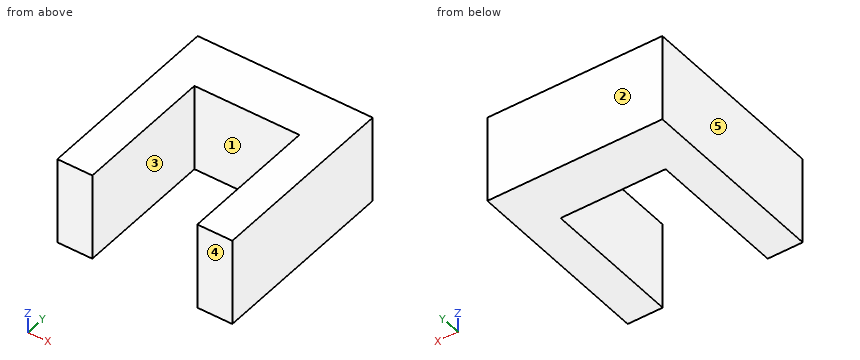
```python
from build123d import *

# Parameters (mm, degrees)
SKETCH1_W           = 50
SKETCH1_H           = 15
BOSS_EXTRUDE1_DEPTH = 25
SKETCH2_W           = 10
SKETCH2_H           = 41
BOSS_EXTRUDE2_DEPTH = 25
SKETCH3_W           = 10
SKETCH3_H           = 41
BOSS_EXTRUDE3_DEPTH = 25


with BuildPart() as part:
    # Sketch1 → Boss-Extrude1 (new body)
    with BuildSketch(Plane.XY):
        with Locations((0, 7.5)):
            Rectangle(SKETCH1_W, SKETCH1_H)
    extrude(amount=BOSS_EXTRUDE1_DEPTH)

    # Sketch2 → Boss-Extrude2 (add)
    with BuildSketch(Plane.XY):
        with Locations((-20, -19.5)):
            Rectangle(SKETCH2_W, SKETCH2_H)
    extrude(amount=BOSS_EXTRUDE2_DEPTH)

    # Sketch3 → Boss-Extrude3 (add)
    with BuildSketch(Plane.XY):
        with Locations((20, -19.5)):
            Rectangle(SKETCH3_W, SKETCH3_H)
    extrude(amount=BOSS_EXTRUDE3_DEPTH)


solid = part.part
```
Work out the finished part from the listing and answer in its coordinate system (mm). Face numbers are marked on the shaded views. A direction names the side the tool comes from. Give positions to 0.01 mm unless a question says otherwise; leave off trailing zeros. Loops run counter-clockwise (first coordinate to the right, second up) from the corner with the lowest first, then second, coordinate; pieces in that order, holes last. Notation, with made-up numbers: (-12.5, 60) - (27.5, 60) arc R9 cw to (27.5, 67) - close; hole circle Ø9 at (8, 5). An arc over 180 degrees is marked (long way). Use CSV: the item, a comma, the result in double quotes. Start each with the question number.
(1) Find section C-C, the plane x = -12. Determine the outline of the cut face in (y, z), plus the area to 3 significant figures.
(2) Find the intervals of material crossed by L1, parallel to X at y = -1.5, z = 18; L2, parallel to Y at x = -9, z = 11.5, in increasing order.
(3) A tool of negligible diameter and unlimited length cuts with its end or side. For the marked faces 1 and 2, from which of +Z, -Z, +X, -X, +Y, -Y can it reach the whole face along a straight path? Write none if from no direction.
(4) Determine the mould class of the marked faces 3, 4 and 5 for opening direction X: released by +X, released by -X, zero draft, split by the parting line, or undercut.
(5) This flat-tipped pin is pushed along its axis until it touches: pin 1 (8 mm diameter, centred on x = -8, z = 15, fed in from -Y). Where does it stop, or does it pass through?
(6) Find section A-A, the plane y = -1.5. Determine the outline of the cut face in (x, z).
(7) Find section B-B, the plane z = 22.75. Determine the outline of the cut face in (x, y).
Results found:
1,outline,"(0, 0) - (15, 0) - (15, 25) - (0, 25) - close"
1,area,"375 mm^2"
2,L1,"-25 to -15, 15 to 25"
2,L2,"0 to 15"
3,face 1,"+Z, -Z, -Y"
3,face 2,"+Z, -Z, +X, -X, +Y"
4,face 3,"undercut"
4,face 4,"zero draft"
4,face 5,"released by -X"
5,pin 1,"y = 0"
6,outline,"(-25, 0) - (-15, 0) - (-15, 25) - (-25, 25) - close; (15, 0) - (25, 0) - (25, 25) - (15, 25) - close"
7,outline,"(-25, -40) - (-15, -40) - (-15, 0) - (15, 0) - (15, -40) - (25, -40) - (25, 15) - (-25, 15) - close"
